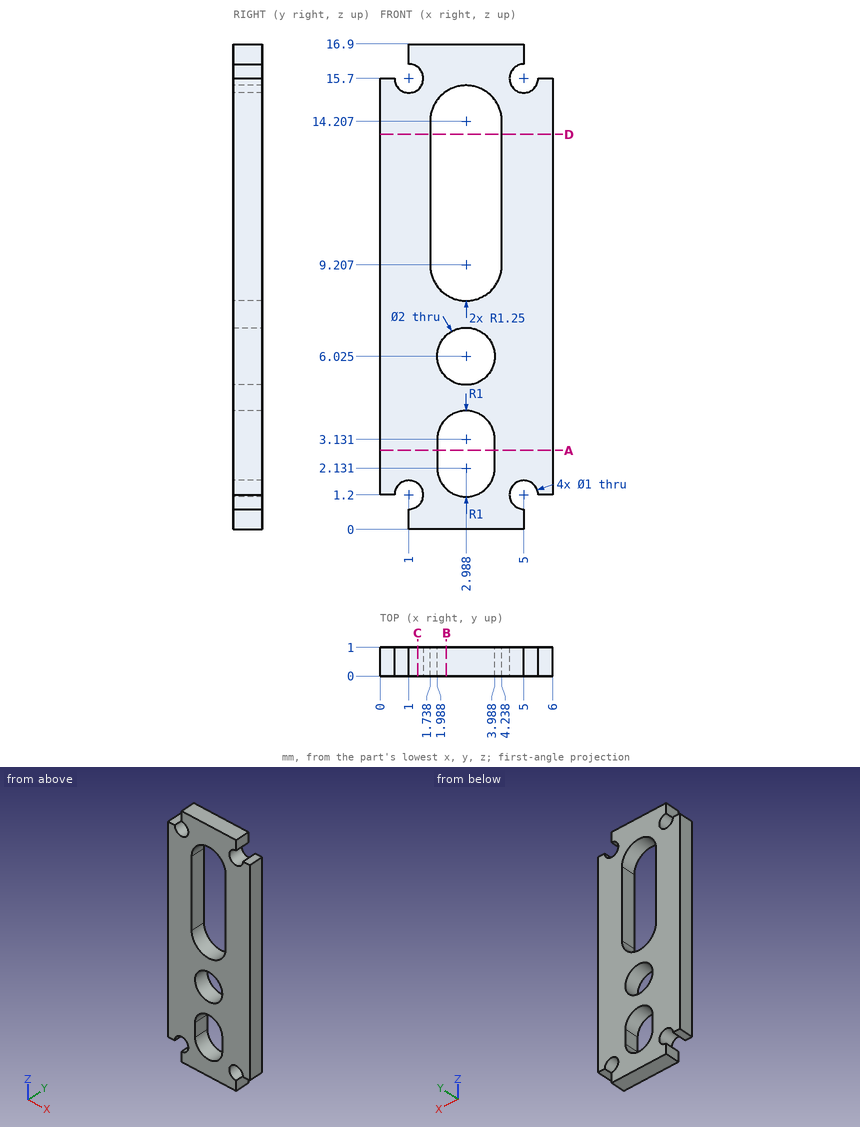
For this review, use the dimensioned drawing (mm, ordinates from the lowest corner) and the shaded views. Give positions to 0.01 mm unless a question says otherwise; leave off trailing zeros. Order: outer loops, then holes, each group sorted by start corner. A loop starts at its lowest first (then second) coordinate and runs counter-clockwise, first axis right, second up. Notation, with made-up numbers: (-32, -32) -> (7, -32) arc R9 cw to (7, -18) -> close; hole circle Ø11 at (83, 39.25). An arc over 180 degrees is marked (long way). Write item = value, one per line. Start each with the question number.
(1) Take a section at D-D (z = 13.75). Write out the cut boundary in (x, y), plus the area to 3 significant figures.
(2) Take a section at C-C (x = 1.3). Write out the cut boundary in (y, z), plus the area to 3 significant figures.
(3) For L1, parallel to X at y = 0.95, z = 10; L2, parallel to X at y = 0.85, z = 1.25 (1 decimal); L3, parallel to Z at x = 3.1, y = 0.4 (1 decimal), list the stretches that pass through material, from the lowest coordinate up. Write a range as from..to.
(4) Take a section at A-A (z = 2.75). Write out the cut boundary in (x, y).
(5) For pin 1 Ø0.8 at (x, z) = (1, 1.2) entering from -Y; pin 2 Ø0.6 at (x, y) = (0, 0.5) entering from +Z; pin 3 Ø1.2 at (x, z) = (5, 1.2) entering from +Y, all flat-tipped, find the tip position at first contact; note any pin that passes through.
(6) Take a section at B-B (x = 2.3). Write out the cut boundary in (y, z).
Returned:
q1.outline = (0, 0) -> (1.74, 0) -> (1.74, 1) -> (0, 1) -> close; (4.24, 0) -> (6, 0) -> (6, 1) -> (4.24, 1) -> close
q1.area = 3.50 mm²
q2.outline = (0, 0) -> (1, 0) -> (1, 0.8) -> (0, 0.8) -> close; (0, 1.6) -> (1, 1.6) -> (1, 15.3) -> (0, 15.3) -> close; (0, 16.1) -> (1, 16.1) -> (1, 16.9) -> (0, 16.9) -> close
q2.area = 15.3 mm²
q3.L1 = 0..1.74, 4.24..6
q3.L2 = 0..0.5, 1.5..2.5, 3.5..4.5, 5.5..6
q3.L3 = 0..1.1, 4.1..5, 7..8, 15.5..16.9
q4.outline = (0, 0) -> (1.99, 0) -> (1.99, 1) -> (0, 1) -> close; (3.99, 0) -> (6, 0) -> (6, 1) -> (3.99, 1) -> close
q5.pin_1 = through
q5.pin_2 = 15.7
q5.pin_3 = 1
q6.outline = (0, 0) -> (1, 0) -> (1, 1.41) -> (0, 1.41) -> close; (0, 3.86) -> (1, 3.86) -> (1, 5.3) -> (0, 5.3) -> close; (0, 6.75) -> (1, 6.75) -> (1, 8.16) -> (0, 8.16) -> close; (0, 15.25) -> (1, 15.25) -> (1, 16.9) -> (0, 16.9) -> close
